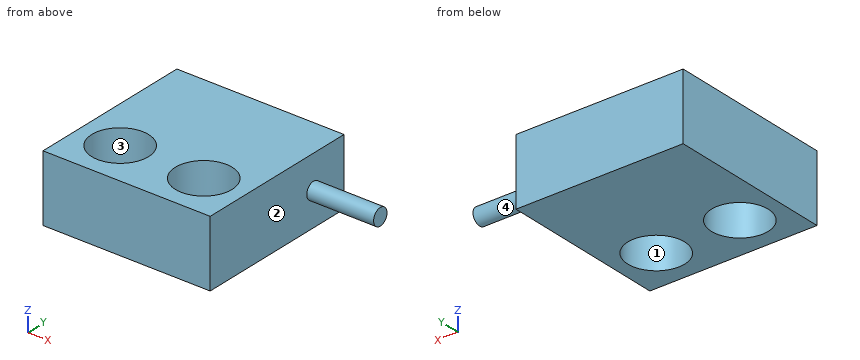
from build123d import *

# Parameters (mm, degrees)
SKETCH7_W           = 50
SKETCH7_H           = 50
SKETCH7_R           = 8.493197323
BOSS_EXTRUDE4_DEPTH = 20
SKETCH8_R           = 2.5
BOSS_EXTRUDE5_DEPTH = 20


with BuildPart() as part:
    # Sketch7 → Boss-Extrude4 (new body)
    with BuildSketch(Plane.XY):
        with Locations((25, 25)):
            Rectangle(SKETCH7_W, SKETCH7_H)
        with Locations((12.5, 13.210183113)):
            Circle(SKETCH7_R, mode=Mode.SUBTRACT)
        with Locations((37.5, 13.210183113)):
            Circle(SKETCH7_R, mode=Mode.SUBTRACT)
    extrude(amount=BOSS_EXTRUDE4_DEPTH)

    # Sketch8 → Boss-Extrude5 (add)
    with BuildSketch(Plane(origin=(50, 0, 0), x_dir=(0, 0, -1), z_dir=(1, 0, 0))):
        with Locations(Location((-10, 38.577958507, 0), (0, 0, 180))):
            Circle(SKETCH8_R)
    extrude(amount=BOSS_EXTRUDE5_DEPTH)


solid = part.part
Input: part model. Units: mm. Frame: model coordinates. Face numbers are marked on the shaded views. Coordinates: 2 decimals unless noted, no trailing zeros. Loops run counter-clockwise (first coordinate to the right, second up) from the corner with the lowest first, then second, coordinate; pieces in that order, holes last.
(1) First-contact query: pin 1 Ø3 at (y, z) = (44.5, 14) entering from -X; pin 2 Ø4 at (y, z) = (10, 3.5) entering from +X; pin 3 Ø3 at (x, z) = (56.5, 13.5) entering from -Y. Flat tips, straight axial feed; report the tip coordinate or a pass-through.
(2) Section B-B on y = 10.5. Return the cut outline in (x, z).
(3) Pull-direction query (Y, two-part tool) for the marked faces 1, 2, 3 and 4; classes: released by +Y, released by -Y, zero draft, split by the parting line, or undercut.
(4) Section A-A on x = 12.5. Return the cut outline in (y, z), then the cut area to 3 significant figures.
(5) Material intervals for probe 1 along X at (y, z) = (19.5, 4.5); probe 2 along X at (y, z) = (14, 3.5); probe 3 along Y at (x, z) = (12.5, 8.5), sorted ascending.
(6) Section D-D on y = 45. Return the cut outline in (x, z).
(7) Section C-C on z = 16. Return the cut outline in (x, y), then the cut area to 3 significant figures.
Data:
1. pin 1: stops at x = 0
1. pin 2: stops at x = 50
1. pin 3: stops at y = 37.08
2. outline: (0, 0) - (4.45, 0) - (4.45, 20) - (0, 20) - close; (20.55, 0) - (29.45, 0) - (29.45, 20) - (20.55, 20) - close; (45.55, 0) - (50, 0) - (50, 20) - (45.55, 20) - close
3. face 1: undercut
3. face 2: zero draft
3. face 3: undercut
3. face 4: split by the parting line
4. outline: (0, 0) - (4.72, 0) - (4.72, 20) - (0, 20) - close; (21.7, 0) - (50, 0) - (50, 20) - (21.7, 20) - close
4. area: 660 mm2
5. probe 1: x = 0 to 6.79, 18.21 to 31.79, 43.21 to 50
5. probe 2: x = 0 to 4.04, 20.96 to 29.04, 45.96 to 50
5. probe 3: y = 0 to 4.72, 21.7 to 50
6. outline: (0, 0) - (50, 0) - (50, 20) - (0, 20) - close
7. outline: (0, 0) - (50, 0) - (50, 50) - (0, 50) - close; hole circle Ø16.99 at (12.5, 13.21); hole circle Ø16.99 at (37.5, 13.21)
7. area: 2,050 mm2
